Check sheet for the modelled part. Datum: model origin and axes. Units: mm. A direction names the side the tool comes from. Round coordinates to 2 decimals unless told otherwise and drop trailing zeros. Order: outer loops, then holes, each group sorted by start corner. A loop starts at its lowest first (then second) coordinate and runs counter-clockwise, first axis right, second up.
(1) Thickness scan on probe 1 along Y at (x, z) = (3.5, -1.75); probe 2 along X at (y, z) = (10, -5.5); probe 3 along X at (y, z) = (13.5, -2.25). Record the ranges inside material, lowest first.
(2) Sectioned sample at C-C, the plane z = 1.25. Enter the section's corners in (x, y).
(3) Sectioned sample at D-D, the plane z = -5.5. Enter the section's corners in (x, y).
(4) Mould release check, pull along X, two halves, no side actions. Record for faces 3 (the cylindrical face through (2.565, 6.235, -0.105)), 4 (the flat face through (-17.34, 21.53, 0.06)), 5 (the flat face through (30.033, 14.515, 0.063)): released by +X, released by -X, zero draft, split by the parting line, or undercut.
(5) Sectioned sample at B-B, the plane x = 4.5. Enter the section's corners in (y, z).
(6) Sectioned sample at A-A, the plane z = -1. Enter the section's corners in (x, y), and give its area (3 significant figures).
(7) Depth check by flat-ended pin: pin 1 (6 mm diameter, centred on y = 14.5, z = -1, fed in from -X); pin 2 (1.5 mm diameter, centred on y = 18.5, z = 4.5, fed in from +X); pin 3 (1 mm diameter, centred on x = -1.5, z = 4.5, fed in from -Y). Enter the tip coordinate at first touch or a pass-through.
(8) Tool access check on faces 1 (the flat face through (23.97, 4.15, 1.77)), 2 (the cylindrical face through (17.22, 6.22, -0.11)). Record the directions out of +Z, -Z, +X, -X, +Y, -Y that give a thin tool (end or side, any length) a straight path to the whole face; none if there is none.
```python
from build123d import *

# Parameters (mm, degrees)
EXTRUDE_1_DEPTH          = 7.5
CUT_EXTRUDE_1_DEPTH      = 41.653128295
CUT_EXTRUDE_1_DEPTH_BACK = 41.653128295
SKETCH_2_R               = 4.1
CUT_EXTRUDE_2_DEPTH      = 46.227204203
CUT_EXTRUDE_2_DEPTH_BACK = 46.227204203
SKETCH_3_R               = 4.1
FILLET_1_R               = 3


with BuildPart() as part:
    # ｽｹｯﾁ1 → ﾎﾞｽ - 押し出し1 (new, symmetric)
    with BuildSketch(Plane.XY):
        Polygon((0, 0), (-19.435028843, 19.435028843), (-15.192388155, 23.67766953), (2.485281374, 6), (17.334523779, 6), (27.941125497, 16.606601718), (32.183766184, 12.363961031), (19.819805153, 0), align=None)
    extrude(amount=EXTRUDE_1_DEPTH, both=True)

    # ｽｹｯﾁ2 → ｶｯﾄ - 押し出し1 (cut, two sides: drawn at the far end of the back side and taken through both)
    with BuildSketch(Plane(origin=(0, 0, 0), x_dir=(0, 0, 1), z_dir=(-0.7071067811865487, -0.7071067811865464, 0)).offset(-CUT_EXTRUDE_1_DEPTH_BACK)):
        with Locations(Location((0, 19.985281374, 0), (0, 0, 270))):
            Circle(SKETCH_2_R)
    extrude(amount=CUT_EXTRUDE_1_DEPTH + CUT_EXTRUDE_1_DEPTH_BACK, mode=Mode.SUBTRACT)

    # ｽｹｯﾁ3 → ｶｯﾄ - 押し出し2 (cut, two sides: drawn at the far end of the back side and taken through both)
    with BuildSketch(Plane(origin=(9.909902577, -9.909902577, 0), x_dir=(0, 0, -1), z_dir=(0.707106781186549, -0.7071067811865461, 0)).offset(-CUT_EXTRUDE_2_DEPTH_BACK)):
        with Locations(Location((0, 24, 0), (0, 0, 90))):
            Circle(SKETCH_3_R)
    extrude(amount=CUT_EXTRUDE_2_DEPTH + CUT_EXTRUDE_2_DEPTH_BACK, mode=Mode.SUBTRACT)

    # ﾌｨﾚｯﾄ1
    fillet_1_edges = [part.edges().sort_by_distance(p)[0] for p in [
        (30.062445841, 14.485281374, -7.5),
        (30.062445841, 14.485281374, 7.5),
        (0, 0, 0),
        (2.485281374, 6, 0),
        (17.334523779, 6, 0),
        (19.819805153, 0, 0),
        (-17.313708499, 21.556349186, 7.5),
        (-17.313708499, 21.556349186, -7.5),
    ]]
    fillet(fillet_1_edges, radius=FILLET_1_R)


solid = part.part
```
Derived:
1. probe 1: y = 0 to 6.01
1. probe 2: x = -10 to -1.51, 21.33 to 29.82
1. probe 3: x = -9.92 to -5.01, 25.29 to 31.05
2. outline: (-19.44, 19.44) - (-16.89, 16.89) - (-12.65, 21.14) - (-15.19, 23.68) - close; (-11.37, 11.37) - (-0.88, 0.88) arc R3 ccw to (1.24, 0) - (18.58, 0) arc R3 ccw to (20.7, 0.88) - (24.12, 4.3) - (19.88, 8.54) - (18.21, 6.88) arc R3 cw to (16.09, 6) - (3.73, 6) arc R3 cw to (1.61, 6.88) - (-7.13, 15.61) - close; (25.4, 14.06) - (29.64, 9.82) - (32.18, 12.36) - (27.94, 16.61) - close
3. outline: (-19.31, 19.31) - (-0.88, 0.88) arc R3 ccw to (1.24, 0) - (18.58, 0) arc R3 ccw to (20.7, 0.88) - (32.06, 12.24) - (27.82, 16.49) - (18.21, 6.88) arc R3 cw to (16.09, 6) - (3.73, 6) arc R3 cw to (1.61, 6.88) - (-15.07, 23.56) - close
4. face 3: undercut
4. face 4: released by -X
4. face 5: released by +X
5. outline: (0, -7.5) - (6, -7.5) - (6, 7.5) - (0, 7.5) - close
6. outline: (-19.44, 19.44) - (-16.94, 16.94) - (-12.7, 21.19) - (-15.19, 23.68) - close; (-11.32, 11.32) - (-0.88, 0.88) arc R3 ccw to (1.24, 0) - (18.58, 0) arc R3 ccw to (20.7, 0.88) - (24.07, 4.25) - (19.83, 8.49) - (18.21, 6.88) arc R3 cw to (16.09, 6) - (3.73, 6) arc R3 cw to (1.61, 6.88) - (-7.08, 15.56) - close; (25.45, 14.11) - (29.69, 9.87) - (32.18, 12.36) - (27.94, 16.61) - close
6. area: 263 mm2
7. pin 1: stops at x = -17.5
7. pin 2: stops at x = -9.26
7. pin 3: stops at y = 1
8. face 1: +Z, -Z, +X, -Y
8. face 2: +Z, -Z, +Y
